```python
from build123d import *

# Parameters (mm, degrees)
F0_W        = 7.9140815362
F0_H        = 1.0166466236
F0_W_2      = 3
F0_H_2      = 1
F0_R        = 4.5
F1_DEPTH    = 3
F2_T1_DEPTH = 3
F2_T3_DEPTH = 28.8894591878
F2_T5_DEPTH = 23.3681675465


# Not quite as in the source:
# - a fillet or chamfer that OpenCascade refuses, or shapes differently, is made with other operations: its cross-section is extruded or revolved along the edge and cut away or added


with BuildPart() as f1:
    # F0 (on Top) → F1 (new body)
    with BuildSketch(Plane.XY):
        Polygon((13.4622063488, -0.5), (14.7628532723, -0.5), (17.7628532723, -0.5), (19.0106034279, -0.5), (19.0106034279, 1.1280798353), (13.4622063488, 1.1280798353), align=None)
        Polygon((10.7628532723, -6.6854998734), (7.292940495, -12.6047210891), (10.2724858996, -13.4541141028), (13.7628532723, -7.5), (13.7628532723, -4.5), (10.7628532723, -4.5), align=None)
        with BuildLine():
            Line((-14.7281754762, 1.7223088071), (-8.4750935815, 3.9539961383))
            add(Edge.make_bspline(
                [(-7.8951590451, 4.8302771503), (-8.2686696422, 4.4379188565), (-8.4750935815, 3.9539961383)],
                knots=[1.3532409109, 1.3532409109, 1.3532409109, 1.9420651459, 1.9420651459, 1.9420651459], degree=2, weights=[1, 0.9569728978, 1]))
            Line((-7.8951590451, 4.8302771503), (-16.1634236574, 7.7945101075))
            Line((-16.1634236574, 7.7945101075), (-21.7940099537, 1.9431159599))
            Line((-21.7940099537, 1.9431159599), (-18.813110888, -14.8382401094))
            Line((-18.813110888, -14.8382401094), (-16.2738263607, -4.4602961279))
            Line((-16.2738263607, -4.4602961279), (-14.7281754762, 1.7223088071))
        make_face()
        Polygon((-4.1330147038, -41.823990643), (-6.7042714065, -44.8882950559), (-0.673970324, -44.8882950559), (-0.673970324, -41.823990643), align=None)
        Polygon((7.292940495, -12.6047210891), (-1.5, -10.0980762114), (4.1472461263, -14.8274837274), (5.7260863187, -15.2775711223), align=None)
        Polygon((33.0707170069, -2.4889647029), (33.0707170069, -3.5056113265), (33.0707170069, -3.9974618703), (36.8696413934, -3.9974618703), (36.8696413934, -2.0199886058), (33.0707170069, -2.0199886058), align=None)
        Polygon((18.2495536771, -36.9809648262), (13.8269943134, -39.3890709971), (15.287962521, -42.0721830228), (19.7105218846, -39.6640768519), align=None)
        with Locations((29.1136762388, -2.9972880147)):
            Rectangle(F0_W, F0_H)
        Polygon((-9.0024047358, -23.0926223927), (-10.5024047358, -25.6906986041), (-1.2683224195, -27.5578969), align=None)
        with BuildLine():
            add(Edge.make_bspline(
                [(-8.4750935815, 3.9539961383), (-9.9447387818, 0.5086849859), (-7.0206677136, 2.6382238069)],
                knots=[1.9420651459, 1.9420651459, 1.9420651459, 4.2160777827, 4.2160777827, 4.2160777827], degree=2, weights=[1, 0.420312788, 1]))
            ThreePointArc((-7.0206677136, 2.6382238069), (-6.5359057109, 3.6785780593), (-5.8980778892, 4.6327828799))
            add(Edge.make_bspline(
                [(-5.8980778892, 4.6327828799), (-5.898901623, 5.1347150622), (-6.2072743134, 5.3597039059)],
                knots=[5.6018784444, 5.6018784444, 5.6018784444, 6.2831853072, 6.2831853072, 6.2831853072], degree=2, weights=[1, 0.9425365533, 1]))
            add(Edge.make_bspline(
                [(-6.2072743134, 5.3597039059), (-6.9059188983, 5.8694352869), (-7.8951590451, 4.8302771503)],
                knots=[0, 0, 0, 1.3532409109, 1.3532409109, 1.3532409109], degree=2, weights=[1, 0.7796933083, 1]))
            add(Edge.make_bspline(
                [(-7.8951590451, 4.8302771503), (-8.2686696422, 4.4379188565), (-8.4750935815, 3.9539961383)],
                knots=[1.3532409109, 1.3532409109, 1.3532409109, 1.9420651459, 1.9420651459, 1.9420651459], degree=2, weights=[1, 0.9569728978, 1]))
        make_face()
        Polygon((8.7628532723, -4.5), (10.7628532723, -4.5), (13.7628532723, -4.5), (16.7579661865, -4.5), (20.2354351463, -4.5), (25.1566354707, -4.5), (25.1566354707, -3.5056113265), (25.1566354707, -2.4889647029), (25.1566354707, -1.5), (22.9422256299, -1.5), (17.7628532723, -1.5), (14.7628532723, -1.5), (8.7628532723, -1.5), align=None)
        with BuildLine():
            Line((20.2354351463, -4.5), (18.0979731586, -8.1462329624))
            add(Edge.make_bspline(
                [(18.0979731586, -8.1462329624), (18.0473234504, -9.0044103563), (18.3297842741, -9.5410849899), (18.6251010746, -10.1915458217)],
                knots=[0, 0, 0, 0, 2.1121478481, 2.1121478481, 2.1121478481, 2.1121478481], degree=3))
            Line((18.6251010746, -10.1915458217), (21.5215887874, -10.1907448843))
            add(Edge.make_bspline(
                [(20.2354351463, -4.5), (20.3352533281, -6.2362966128), (20.3635003418, -8.2417670637), (21.5215887874, -10.1907448843)],
                knots=[0, 0, 0, 0, 5.8342753215, 5.8342753215, 5.8342753215, 5.8342753215], degree=3))
        make_face()
        with BuildLine():
            ThreePointArc((0, -7.5), (-1.5760318318, -7.3325386917), (-3.0816838363, -6.8376329774))
            Line((-3.0816838363, -6.8376329774), (-13.1004809472, -24.1906986041))
            Line((-13.1004809472, -24.1906986041), (-10.5024047358, -25.6906986041))
            Line((-10.5024047358, -25.6906986041), (-9.0024047358, -23.0926223927))
            Line((-9.0024047358, -23.0926223927), (-3.0228838472, -12.7357884087))
            Line((-3.0228838472, -12.7357884087), (-1.5, -10.0980762114))
            Line((-1.5, -10.0980762114), (0, -7.5))
        make_face()
        with BuildLine():
            ThreePointArc((-5.8980778892, 4.6327828799), (-6.5359057109, 3.6785780593), (-7.0206677136, 2.6382238069))
            add(Edge.make_bspline(
                [(-7.0206677136, 2.6382238069), (-5.896148589, 3.4571871888), (-5.8980778892, 4.6327828799)],
                knots=[4.2160777827, 4.2160777827, 4.2160777827, 5.6018784444, 5.6018784444, 5.6018784444], degree=2, weights=[1, 0.7693966053, 1]))
        make_face()
        Polygon((11.3319195864, -13.7561318437), (10.2724858996, -13.4541141028), (8.7056317233, -16.1269641361), (12.7446108147, -17.2783748907), (18.0979731586, -8.1462329624), (20.2354351463, -4.5), (16.7579661865, -4.5), align=None)
        Polygon((7.8259082511, -8.0615244806), (10.7628532723, -4.5), (8.7628532723, -4.5), (8.7628532723, -1.5), (7.8259082511, -1.5), align=None)
        with Locations((16.2628532723, -1)):
            Rectangle(F0_W_2, F0_H_2)
        with BuildLine():
            ThreePointArc((-7.0206677136, 2.6382238069), (-6.9254849764, -2.8788292484), (-3.0816838363, -6.8376329774))
            ThreePointArc((-3.0816838363, -6.8376329774), (-1.5760318318, -7.3325386917), (0, -7.5))
            ThreePointArc((0, -7.5), (5.3033008589, -5.3033008589), (7.5, 0))
            ThreePointArc((7.5, 0), (2.4509606107, 7.088215014), (-5.8980778892, 4.6327828799))
            add(Edge.make_bspline(
                [(-7.0206677136, 2.6382238069), (-5.896148589, 3.4571871888), (-5.8980778892, 4.6327828799)],
                knots=[4.2160777827, 4.2160777827, 4.2160777827, 5.6018784444, 5.6018784444, 5.6018784444], degree=2, weights=[1, 0.7693966053, 1]))
        make_face()
        Circle(F0_R, mode=Mode.SUBTRACT)
        Polygon((-1.2683224195, -27.5578969), (-10.5024047358, -25.6906986041), (0.2696389092, -31.9099409022), (-9.0024047358, -42.9599322269), (-6.7042714065, -44.8882950559), (-4.1330147038, -41.823990643), (4.8659055679, -31.0994950798), align=None)
        Polygon((10.2724858996, -13.4541141028), (7.292940495, -12.6047210891), (5.7260863187, -15.2775711223), (8.7056317233, -16.1269641361), align=None)
        Polygon((22.9422256299, -0.2355174292), (22.9422256299, -1.5), (25.1566354707, -1.5), align=None)
        Polygon((6.6801939907, -26.2637573918), (-9.0024047358, -23.0926223927), (-1.2683224195, -27.5578969), (4.616944438, -28.7479404659), (12.6532249158, -43.5068111111), (15.287962521, -42.0721830228), (13.8269943134, -39.3890709971), align=None)
        Polygon((4.1472461263, -14.8274837274), (-1.5, -10.0980762114), (-3.0228838472, -12.7357884087), (6.1770209488, -20.4404462041), (8.7056317233, -16.1269641361), (5.7260863187, -15.2775711223), (5.3831728236, -15.8625370756), align=None)
    extrude(amount=F1_DEPTH)

    # F2: fillet of radius 8 on 3 edges, made by hand

    # F2_s2 → F2_t1 (join)
    with BuildSketch(Plane.XY):
        with BuildLine():
            ThreePointArc((-15.7668598362, -2.4324295718), (-13.9323879929, 1.0007952454), (-10.6947478435, 3.1618148779))
            Line((-10.6947478435, 3.1618148779), (-14.7281754762, 1.7223088071))
            Line((-14.7281754762, 1.7223088071), (-15.7668598362, -2.4324295718))
        make_face()
    extrude(amount=F2_T1_DEPTH)

    # F2_s4 → F2_t3 (cut)
    with BuildSketch(Plane.XY.offset(-12.9447295939)):
        with BuildLine():
            ThreePointArc((-11.2892959012, 6.0470998817), (-15.8144489693, 6.3053971181), (-19.7536720515, 4.0634673109))
            Line((-19.7536720515, 4.0634673109), (-16.1634236574, 7.7945101075))
            Line((-16.1634236574, 7.7945101075), (-11.2892959012, 6.0470998817))
        make_face()
    extrude(amount=F2_T3_DEPTH, mode=Mode.SUBTRACT)

    # F2_s6 → F2_t5 (cut)
    with BuildSketch(Plane.XY.offset(-10.1840837733)):
        with BuildLine():
            ThreePointArc((-18.9694325729, 4.8784613548), (-20.8588428617, 1.6587603608), (-21.0815566526, -2.0677318634))
            Line((-21.0815566526, -2.0677318634), (-21.7940099537, 1.9431159599))
            Line((-21.7940099537, 1.9431159599), (-18.9694325729, 4.8784613548))
        make_face()
    extrude(amount=F2_T5_DEPTH, mode=Mode.SUBTRACT)


solid = f1.part
```
Geometry check sheet. Reference: the model listing, model coordinates, mm. A direction names the side the tool comes from. Give positions to 0.01 mm unless a question says otherwise; leave off trailing zeros. Order: outer loops, then holes, each group sorted by start corner. A loop starts at its lowest first (then second) coordinate and runs counter-clockwise, first axis right, second up. Notation, with made-up numbers: (34.25, -1) - (90.25, -1) arc R16 ccw to (90.25, 20) - close; hole circle Ø1 at (-28.75, 82). An arc over 180 degrees is marked (long way). Write item = value, one per line. Start each with the question number.
1) Section check A-A (y = -11). Enter the section's corners in (x, z), then the cut area to 3 significant figures.
2) Section check B-B (z = 2.3). Count the separate pieces of the cut face and the enclosed holes in it, then the cut area to 3 significant figures.
3) Gauge pin test, flat ends, axial feed: pin 1 Ø0.8 at (y, z) = (-1, 2) entering from +X; pin 2 Ø1.5 at (x, z) = (16.5, 2) entering from +Y; pin 3 Ø0.8 at (y, z) = (0.5, 2) entering from -X. Record the tip position at first contact, or that the pin passes through.
4) Scan lines: L1, parallel to Y at x = 0, z = 0.9; L2, parallel to Y at x = -8, z = 1.95; L3, parallel to Y at x = 16, z = 2.6. Record each from-to range of solid material in increasing order.
5) Access from +Z, -Z, +X, -X, +Y, -Y to the whole of each face (thin tool, end or side, straight path). Record for faces 4 (the flat face through (7.826, -5, 1)), 5 (the flat face through (11, -1.5, 1)), 6 (the flat face through (-16.024, -3.461, 1.479)).
6) Draft check along X on faces 1 (the flat face through (2.96, -11.37, 1.48)), 2 (the flat face through (16, 1.128, 1)), 3 (the flat face through (-1.05, -24.7, 1.48)). Enter one of: released by +X, released by -X, zero draft, split by the parting line, or undercut.
Geometry check:
q1.outline = (-19.49, 0) - (-17.87, 0) - (-17.87, 3) - (-19.49, 3) - close; (-5.48, 0) - (1.66, 0) - (1.66, 3) - (-5.48, 3) - close; (8.23, 0) - (11.71, 0) - (11.71, 3) - (8.23, 3) - close; (12.95, 0) - (16.43, 0) - (16.43, 3) - (12.95, 3) - close
q1.area = 47.2 mm2
q2.separate_pieces = 1
q2.enclosed_holes = 3
q2.area = 722 mm2
q3.pin_1 = 24.98
q3.pin_2 = 1.13
q3.pin_3 = -21.17
q4.L1 = -36.9 to -32.23, -31.75 to -28.29, -27.81 to -24.91, -15.27 to -10.53, -7.5 to -4.5, 4.5 to 7.5
q4.L2 = -43.8 to -41.77, -27.14 to -23.3, -21.36 to -15.36, 2.3 to 4.87
q4.L3 = -41.68 to -38.21, -11.73 to -5.79, -4.5 to 1.13
q5.face_4 = +Z, -Z, +Y
q5.face_5 = +Z, -Z
q5.face_6 = +Z, -Z, -Y
q6.face_1 = undercut
q6.face_2 = zero draft
q6.face_3 = released by +X
